Autodesk Fusion 360 part; units mm, degrees
sketch "Hub" plane through (0, 0, 0) normal (0, 1, 0) x (1, 0, 0)
  circle A0 centre (0, 0) radius 8.89
  dimension "d8" = 17.78
extrude "Extrude1" add sketch "Hub" along normal blind 15.24
sketch "Inner Cap" plane through (0, 0, 0) normal (0, -1, 0) x (1, 0, 0)
  circle A0 centre (0, 0) radius 8.89
  circle A1 centre (0, 0) radius 9.7155
  dimension "d11" = 19.431
extrude "Extrude2" add sketch "Inner Cap" against normal blind 1.27 contours A0 | A1
sketch "Outer Cap" plane through (0, 15.24, 0) normal (0, 1, 0) x (-1, 0, 0)
  circle A0 centre (0, 0) radius 8.89
  circle A1 centre (0, 0) radius 9.7155
  circle A2 centre (0, 0) radius 9.7155
  circle A3 centre (0, 0) radius 9.7155
extrude "Extrude3" add sketch "Outer Cap" against normal blind 1.27 contours A0 | A1 A2 A3
sketch "Bore" plane through (0, 15.24, 0) normal (0, 1, 0) x (-1, 0, 0)
  circle A0 centre (0, 0) radius 9.7155
  circle A1 centre (0, 0) radius 4.191
  dimension "d16" = 8.382
extrude "Extrude4" cut sketch "Bore" against normal blind 12.065 contours A1
sketch "Screw Hole" plane through (0, 15.24, 0) normal (0, 1, 0) x (-1, 0, 0)
  circle A0 centre (0, 0) radius 1.524
  dimension "d19" = 3.048
extrude "Extrude5" cut sketch "Screw Hole" against normal blind 72.644
equation "hubDia = 0.7 in"
equation "boreDia = 0.33 in"
equation "boreDepth = 0.475 in"
equation "screwHole = 0.12 in"
equation "capEndDia = 0.765 in"
equation "capThickness = 0.05 in"
equation "d8 = hubDia"
equation "d11 = capEndDia"
equation "d16 = boreDia"
equation "d19 = screwHole"
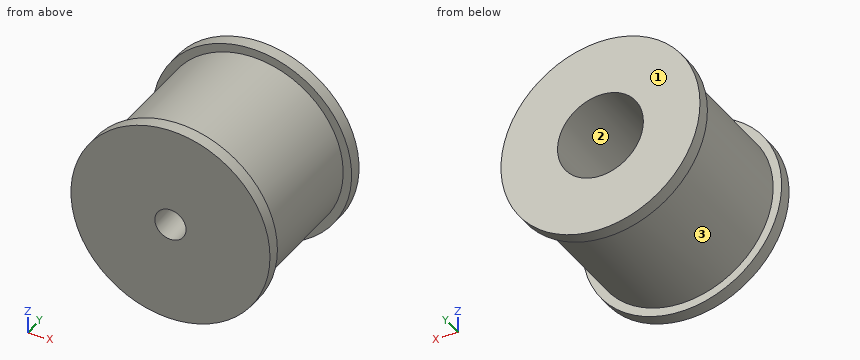
Check sheet for the modelled part. Datum: model origin and axes. Units: mm. Face numbers are marked on the shaded views. Round coordinates to 2 decimals unless told otherwise and drop trailing zeros. Order: outer loops, then holes, each group sorted by start corner. A loop starts at its lowest first (then second) coordinate and runs counter-clockwise, first axis right, second up.
(1) Draft check along Z on the marked faces 1, 2 and 3. Enter one of: pulls with the +Z half, pulls with the -Z half, needs draft (parallel to the pull), parting line crosses it, or undercut.
(2) Cross-section at A-A, the plane z = 0. Enter the section's corners in (x, y) (1 decimal), and give its area (3 significant figures).
(3) Cross-section at D-D, the plane x = -7.5. Enter the section's corners in (y, z), and give its area (3 significant figures).
(4) Scan lines: probe 1 along Z at (x, y) = (0, 2.3); probe 2 along Z at (x, y) = (0, 9); probe 3 along Y at (x, z) = (-4, 0.75) (3 decimals). Record each from-to range of solid material in increasing order.
(5) Go/stop test with flat-tipped pins: P1, Ø1, axis at y = 7.5, z = 1.5, coming from the +X side; P2, Ø2.5, axis at x = 2, z = 2, coming from the +Y side (3 decimals); P3, Ø6, axis at y = 9, z = -1.5, coming from the -X side. Record where each tip stops, or that it passes through.
(6) Cross-section at C-C, the plane y = 2.25. Enter the section's corners in (x, z).
(7) Cross-section at B-B, the plane x = 0. Enter the section's corners in (y, z) (1 decimal).
Check sheet entries:
1. face 1: needs draft
1. face 2: undercut
1. face 3: parting line crosses it
2. outline: (-9.7, 0) - (-1.5, 0) - (-1.5, 3.2) - (-4.2, 3.2) - (-4.2, 15.2) - (-9.7, 15.2) - (-9.7, 14) - (-8.9, 14) - (-8.9, 1.3) - (-9.7, 1.3) - close; (1.5, 0) - (9.7, 0) - (9.7, 1.3) - (8.9, 1.3) - (8.9, 14) - (9.7, 14) - (9.7, 15.2) - (4.2, 15.2) - (4.2, 3.2) - (1.5, 3.2) - close
2. area: 164 mm2
3. outline: (0, -6.18) - (1.27, -6.18) - (1.27, -4.77) - (13.97, -4.77) - (13.97, -6.18) - (15.24, -6.18) - (15.24, 6.18) - (13.97, 6.18) - (13.97, 4.77) - (1.27, 4.77) - (1.27, 6.18) - (0, 6.18) - close
3. area: 153 mm2
4. probe 1: z = -8.89 to -1.52, 1.52 to 8.89
4. probe 2: z = -8.89 to -4.19, 4.19 to 8.89
4. probe 3: y = 0 to 3.175
5. P1: stops at x = 8.83
5. P2: stops at y = 3.175
5. P3: stops at x = -8.89
6. outline: circle Ø17.78 at (0, 0); hole circle Ø3.05 at (0, 0)
7. outline: (0, -9.7) - (1.3, -9.7) - (1.3, -8.9) - (14, -8.9) - (14, -9.7) - (15.2, -9.7) - (15.2, -4.2) - (3.2, -4.2) - (3.2, -1.5) - (0, -1.5) - close; (0, 1.5) - (3.2, 1.5) - (3.2, 4.2) - (15.2, 4.2) - (15.2, 9.7) - (14, 9.7) - (14, 8.9) - (1.3, 8.9) - (1.3, 9.7) - (0, 9.7) - close
